Check sheet for the drawn part. Datum: minimum x, y, z corner. Units: mm. A direction names the side the tool comes from. Coordinates: 2 decimals unless noted, no trailing zeros. Loops run counter-clockwise (first coordinate to the right, second up) from the corner with the lowest first, then second, coordinate; pieces in that order, holes last. Notation, with made-up numbers: M -39.5,-26 L -21.5,-26 A19 cw -21.5,-22 Z; hole C 1,-3 d3. An arc over 180 degrees is marked long. Use CSV: the item, a comma, the result in double quotes. Start each with the question number.
(1) Section check A-A on x = 103. Record the cut outline in (y, z).
(2) Draft check along X on the marked faces 4, 5, 6 and 7. Enter one of: pulls with the +X half, pulls with the -X half, needs draft (parallel to the pull), parting line crosses it, or undercut.
(3) Section check B-B on z = 22.75. Record the cut outline in (x, y).
(4) Go/stop test with a flat-tipped pin: pin 1 Ø7 at (x, z) = (76.5, 19.5) entering from -Y. Record where the tip stops, or that it passes through.
(5) Section check D-D on z = 8.75. Record the cut outline in (x, y).
(6) Set-up check for the marked faces 1, 2 and 3: record each of +Z, -Z, +X, -X, +Y, -Y from which the full face is reachable in a straight line by a thin tool's end or side.
(7) Section check C-C on y = 38. Record the cut outline in (x, z).
(8) Scan lines: line 1 (Y direction, x = 61, z = 5.5); line 2 (X direction, y = 80.5, z = 17.5); line 3 (Z direction, x = 75, y = 73.5). Record each from-to range of solid material in increasing order.
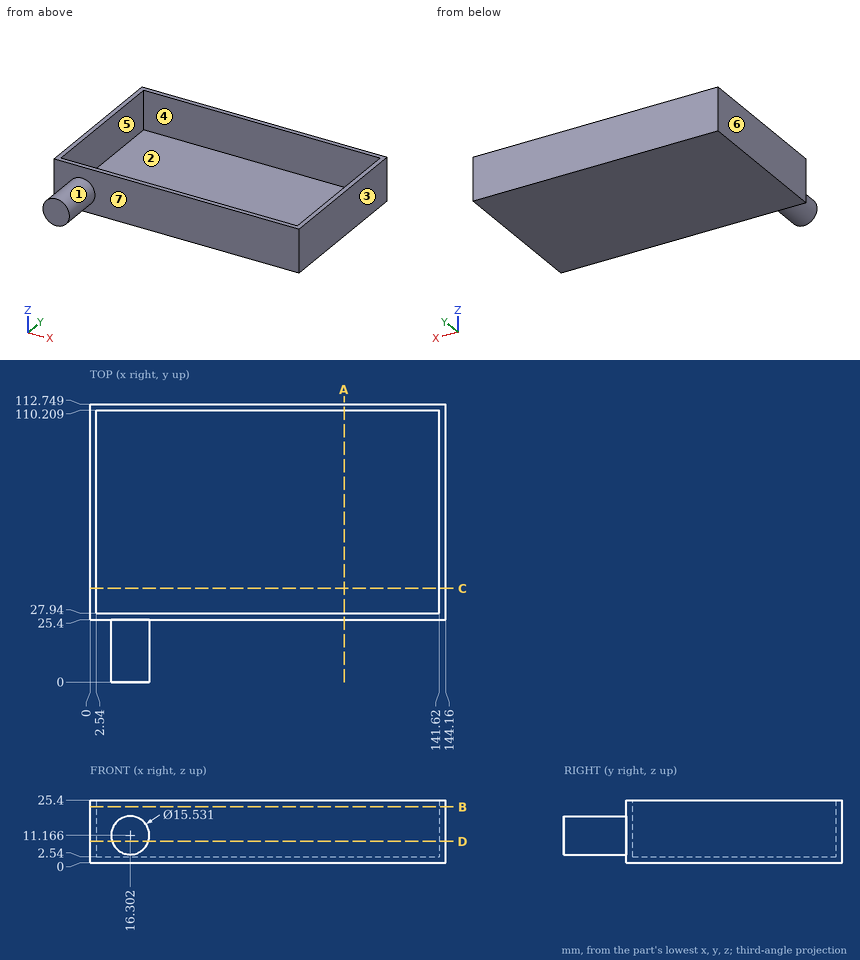
Outcome:
1,outline,"M 25.4,0 L 112.75,0 L 112.75,25.4 L 110.21,25.4 L 110.21,2.54 L 27.94,2.54 L 27.94,25.4 L 25.4,25.4 Z"
2,face 4,"undercut"
2,face 5,"undercut"
2,face 6,"pulls with the -X half"
2,face 7,"needs draft"
3,outline,"M 0,25.4 L 144.16,25.4 L 144.16,112.75 L 0,112.75 Z; hole M 2.54,27.94 L 141.62,27.94 L 141.62,110.21 L 2.54,110.21 Z"
4,pin 1,"stops at y = 25.4"
5,outline,"M 0,25.4 L 8.92,25.4 L 8.92,0 L 23.68,0 L 23.68,25.4 L 144.16,25.4 L 144.16,112.75 L 0,112.75 Z; hole M 2.54,27.94 L 141.62,27.94 L 141.62,110.21 L 2.54,110.21 Z"
6,face 1,"-Y"
6,face 2,"+Z"
6,face 3,"+Z, -Z, +X, +Y, -Y"
7,outline,"M 0,0 L 144.16,0 L 144.16,25.4 L 141.62,25.4 L 141.62,2.54 L 2.54,2.54 L 2.54,25.4 L 0,25.4 Z"
8,line 1,"y = 25.4 to 27.94, 110.21 to 112.75"
8,line 2,"x = 0 to 2.54, 141.62 to 144.16"
8,line 3,"z = 0 to 2.54"
